from build123d import *

# Parameters (mm, degrees)
F1_DEPTH = 76.2
F2_R     = 5.08
F3_R     = 5.08
F5_D     = 25.4


with BuildPart() as f1:
    # F0 (on Front) → F1 (new body)
    with BuildSketch(Plane.XZ):
        Polygon((12.929662, 52.085873), (-61.460182, 56.824941), (-44.102553, 27.828874), (0, 20.160461), align=None)
    extrude(amount=-F1_DEPTH)

    # F2
    f2_edges = [f1.edges().sort_by_distance(p)[0] for p in [
        (-24.26526, 0, 54.455407),
    ]]
    fillet(f2_edges, radius=F2_R)

    # F3
    f3_edges = [f1.edges().sort_by_distance(p)[0] for p in [
        (-22.051277, 0, 23.994667),
    ]]
    fillet(f3_edges, radius=F3_R)

    # F5 (through all)
    with Locations(Plane(origin=(3.357025, 0, 52.695706), x_dir=(0.997977, 0, -0.063577), z_dir=(0.063577, 0, 0.997977))):
        with Locations((-30.832324, 41.9522)):
            Hole(F5_D / 2)


solid = f1.part
Work out the finished part from the listing and answer in its coordinate system (mm). Round coordinates to 2 decimals unless told otherwise and drop trailing zeros. Write each loop counter-clockwise with the first axis right and the second up, starting at its lowest first coordinate (ties: lowest second). Pieces come first, ordered by that corner, then holes.
1) A cutting plane is placed at A-A (y = 31.5). Give the vertices of the cut face in (x, z).
2) A cutting plane is placed at B-B (y = 57). Give the vertices of the cut face in (x, z).
3) Straight lines are drawn through the part: line 1 (X direction, y = 45.5, z = 50.5); line 2 (X direction, y = 41.5, z = 40); line 3 (X direction, y = 13.5, z = 28.5). For each, find the intervals that lie inside material, in ascending order.
4) The mould has two halves that part along X. Classify faces 1 (the cylindrical face through (-15.75, 42.51, 38.18)), 2 (the flat face through (-25, 76.2, 39)), 3 (the flat face through (-12.559, 40.142, 22.344)), 4 (the flat face through (-15.479, 32.24, 53.896)): pulls with the +X half, pulls with the -X half, needs draft (parallel to the pull), parting line crosses it, or undercut.
5) Given pin 1 Ø3 at (y, z) = (59.5, 28) entering from -X; pin 2 Ø5 at (y, z) = (13, 49.5) entering from -X; pin 3 Ø10 at (x, y) = (-30.5, 46) entering from -Z; pin 4 Ø12 at (y, z) = (68.5, 37.5) entering from +X, each flat-ended and moving along its own axis, determine where each tip first touches the part or whether it passes through.
Completed:
1. outline: (-61.46, 56.82) - (-44.1, 27.83) - (-36.44, 26.5) - (-34.61, 55.11) - close; (-22.14, 24.01) - (0, 20.16) - (12.93, 52.09) - (-20.21, 54.2) - close
2. outline: (-61.46, 56.82) - (-44.1, 27.83) - (0, 20.16) - (12.93, 52.09) - close
3. line 1: x = -57.67 to -39.9, -15.46 to 12.29
3. line 2: x = -51.39 to -41.06, -15.63 to 8.03
3. line 3: x = -44.5 to 3.38
4. face 1: undercut
4. face 2: needs draft
4. face 3: pulls with the -X half
4. face 4: pulls with the +X half
5. pin 1: stops at x = -45.1
5. pin 2: stops at x = -58.57
5. pin 3: passes through
5. pin 4: stops at x = 9.45
